Can you work these out from the model? Positions are in its coordinate system, mm. Coordinates: 2 decimals unless noted, no trailing zeros. Order: outer loops, then holes, each group sorted by start corner. A loop starts at its lowest first (then second) coordinate and runs counter-clockwise, first axis right, second up. Notation, with made-up numbers: (5.5, 60) -> (9.5, 60) arc R34 cw to (9.5, 94) -> close; hole circle Ø10 at (-10.5, -26.5). An arc over 180 degrees is marked (long way). Answer in a Markdown table with one row per item.
```python
from build123d import *

# Parameters (mm, degrees)
SKETCH1_R                      = 3.175
BOSS_EXTRUDE1_DEPTH            = 2.54
DOME1_FACE_RADIUS              = 3.175
DOME1_HEIGHT                   = 25.4
SKETCH8_R                      = 1.5875
CUT_EXTRUDE1_DEPTH             = 6.35
F_4_0_209_DIAMETER_HOLE1_D     = 5.3086
F_4_0_209_DIAMETER_HOLE1_DEPTH = 6.35
F_4_0_209_DIAMETER_HOLE1_TIP   = 1.594864341


with BuildPart() as part:
    # Sketch1 → Boss-Extrude1 (new body)
    with BuildSketch(Plane(origin=(0, 0, 0), x_dir=(1, 0, 0), z_dir=(0, 1, 0))):
        with Locations(Location((0, 0, 0), (0, 0, 270))):
            Circle(SKETCH1_R)
    extrude(amount=BOSS_EXTRUDE1_DEPTH)

    # Dome1: a dome of height H over a round flat face of radius A is a cap of a sphere of radius (A * A + H * H) / (2 * H)
    dome1_r = (DOME1_FACE_RADIUS * DOME1_FACE_RADIUS + DOME1_HEIGHT * DOME1_HEIGHT) / (2 * DOME1_HEIGHT)
    dome1_base = Plane((0, 2.54, 0), z_dir=(0, 1, 0))
    with Locations(dome1_base.offset(DOME1_HEIGHT - dome1_r)):
        dome1_ball = Sphere(dome1_r, mode=Mode.PRIVATE)
    add(split(dome1_ball, bisect_by=dome1_base, keep=Keep.TOP, mode=Mode.PRIVATE))

    # Sketch8 → Cut-Extrude1 (cut)
    with BuildSketch(Plane.XZ):
        with Locations(Location((0, 0, 0), (0, 0, 270))):
            Circle(SKETCH8_R)
    extrude(amount=-CUT_EXTRUDE1_DEPTH, mode=Mode.SUBTRACT)

    # #4 (0.209) Diameter Hole1
    with Locations(Plane(origin=(0, 0, 0), x_dir=(-1, 0, 0), z_dir=(0, -1, 0))):
        with Locations((0, 0)):
            Hole(F_4_0_209_DIAMETER_HOLE1_D / 2, depth=F_4_0_209_DIAMETER_HOLE1_DEPTH)
            with Locations((0, 0, -(F_4_0_209_DIAMETER_HOLE1_DEPTH + F_4_0_209_DIAMETER_HOLE1_TIP / 2))):  # 118° drill point
                Cone(0, F_4_0_209_DIAMETER_HOLE1_D / 2, F_4_0_209_DIAMETER_HOLE1_TIP, mode=Mode.SUBTRACT)


solid = part.part
```
(1) Suppose I cut it at A-A (z = -6.5). Please give me the cut outline in (x, y), and give its area (3 significant figures).
Response values:
| item | result |
|---|---|
| outline | circle Ø22.28 at (0, 15.04) |
| area | 390 mm2 |
(2) Suppose I cut it at C-C (y = 7). Please give me the cut outline in (x, z), and give its area (3 significant figures).
Response values:
| item | result |
|---|---|
| outline | circle Ø20.17 at (0, 0); hole circle Ø3.15 at (0, 0) |
| area | 312 mm2 |
(3) Will these pins go through, and if not, where does the flat tip stop? pin 1 Ø5 at (y, z) = (13.5, 9) entering from -X; pin 2 Ø10 at (x, y) = (6.5, 11) entering from +Z; pin 3 Ø6 at (x, z) = (-9.5, -4) entering from +Y.
Response values:
| item | result |
|---|---|
| pin 1 | x = -11.06 |
| pin 2 | z = 12.62 |
| pin 3 | y = 25.67 |
(4) Suppose I cut it at B-B (y = 10.25). Please give me the cut outline in (x, z).
Response values:
| item | result |
|---|---|
| outline | circle Ø23.95 at (0, 0) |
(5) We'd pull the mould along X, two halves only. Please class faces 1 (the cylindrical face through (-1.93, 1.25, -2.52)), 2 (the flat face through (-2, 0, 2)), 3 (the conical face through (0.1, 7.67, 0.45)): +X half, -X half, draft (parallel to the pull), parting line (faces both ways), or undercut.
Response values:
| item | result |
|---|---|
| face 1 | parting line |
| face 2 | draft |
| face 3 | undercut |
(6) I need wall thicknesses on line 1 (Z direction, x = 1.5, y = 4); line 2 (Y direction, x = -3, z = -8.25); line 3 (Z direction, x = -1, y = 14). Which ranges of each line are inside material? Lowest first, please. Write a range as [from, to].
Response values:
| item | result |
|---|---|
| line 1 | [-6.5, -2.19], [2.19, 6.5] |
| line 2 | [5.59, 24.49] |
| line 3 | [-12.82, 12.82] |
